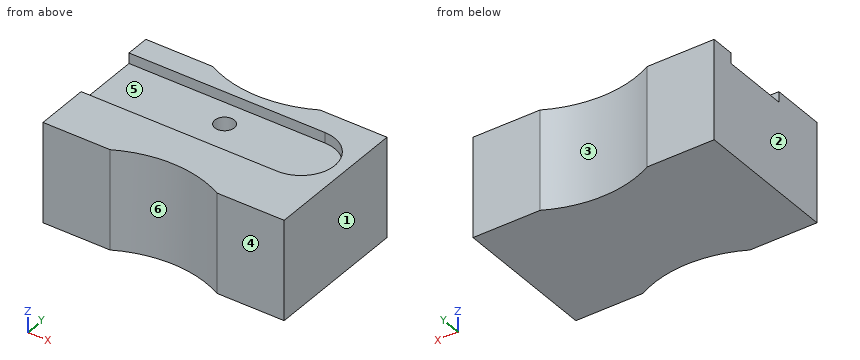
from build123d import *

# Parameters (mm, degrees)
F1_DEPTH = 10.5
F2_DEPTH = 1.1
F3_R     = 1.025
F4_DEPTH = 2.5


with BuildPart() as f1:
    # F0 (on Top) → F1 (new body)
    with BuildSketch(Plane.XY):
        with BuildLine():
            Line((-7.05, 0), (0, 0))
            Line((0, 0), (0, 15.25))
            Line((0, 15.25), (-7.05, 15.25))
            ThreePointArc((-7.05, 15.25), (-12.675, 13.856541), (-18.3, 15.25))
            Line((-18.3, 15.25), (-25.35, 15.25))
            Line((-25.35, 15.25), (-25.35, 12.75))
            Line((-25.35, 12.75), (-4.75, 12.75))
            ThreePointArc((-4.75, 12.75), (-1.2, 9.2), (-4.75, 5.65))
            Line((-4.75, 5.65), (-25.35, 5.65))
            Line((-25.35, 5.65), (-25.35, 0))
            Line((-25.35, 0), (-18.3, 0))
            ThreePointArc((-18.3, 0), (-12.675, 1.393459), (-7.05, 0))
        make_face()
        with BuildLine():
            Line((-25.35, 12.75), (-25.35, 5.65))
            Line((-25.35, 5.65), (-4.75, 5.65))
            ThreePointArc((-4.75, 5.65), (-1.2, 9.2), (-4.75, 12.75))
            Line((-4.75, 12.75), (-25.35, 12.75))
        make_face()
    extrude(amount=-F1_DEPTH)

    # F0 (on Top) → F2 (cut)
    with BuildSketch(Plane.XY):
        with BuildLine():
            Line((-25.35, 12.75), (-25.35, 5.65))
            Line((-25.35, 5.65), (-4.75, 5.65))
            ThreePointArc((-4.75, 5.65), (-1.2, 9.2), (-4.75, 12.75))
            Line((-4.75, 12.75), (-25.35, 12.75))
        make_face()
    extrude(amount=-F2_DEPTH, mode=Mode.SUBTRACT)

    # F3 (on face) → F4 (cut)
    with BuildSketch(Plane.XY.offset(-1.1)):
        with Locations((-13.425, 10.1)):
            Circle(F3_R)
    extrude(amount=-F4_DEPTH, mode=Mode.SUBTRACT)


solid = f1.part
Work out the finished part from the listing and answer in its coordinate system (mm). Face numbers are marked on the shaded views. A direction names the side the tool comes from. Give positions to 0.01 mm unless a question says otherwise; leave off trailing zeros. Loops run counter-clockwise (first coordinate to the right, second up) from the corner with the lowest first, then second, coordinate; pieces in that order, holes last. Notation, with made-up numbers: (48.25, -39) - (82.25, -39) arc R23 cw to (82.25, -19) - close; hole circle Ø7 at (67.5, 77.5). An arc over 180 degrees is marked (long way). Answer in a Markdown table with one row per item. Add a question column.
Q1. The part is cut by section C-C (z = -8.25). Determine the outline of the cut face in (x, y) (3 decimals).
Q2. Consider line 1 along Y through (x, z) = (-6.25, -1); line 2 along Z through (x, y) = (-12.5, 7.5); line 3 along Y through (x, z) = (-12.5, -2.25). Determine where each line is inside the solid, lowest interval first.
Q3. The part is cut by section A-A (z = -2.5). Determine the outline of the cut face in (x, y) (3 decimals), and give its area (3 significant figures).
Q4. Each of these flat-tipped pins is pushed along its axis until it touches: P1, Ø0.6, axis at x = -12, z = -0.5, coming from the +Y side; P2, Ø2, axis at x = -10.5, y = 9, coming from the +Z side; P3, Ø6, axis at x = -13, z = -5, coming from the -Y side. Where does it stop, or does it pass through?
Q5. The part is cut by section B-B (x = -18.75). Determine the outline of the cut face in (y, z), and give its area (3 significant figures).
Q6. The part is cut by section D-D (y = 9.5). Determine the outline of the cut face in (x, z).
Q7. A tool of negligible diameter and unlimited length cuts with its end or side. For the marked faces 5 and 6, from which of +Z, -Z, +X, -X, +Y, -Y can it reach the whole face along a straight path? Write none if from no direction.
Q8. Determine the mould class of the marked faces 1, 2, 3 and 4 for opening direction X: released by +X, released by -X, zero draft, split by the parting line, or undercut.
Solution:
| question | item | result |
|---|---|---|
| 1 | outline | (-25.35, 0) - (-18.3, 0) arc R12.05 cw to (-7.05, 0) - (0, 0) - (0, 15.25) - (-7.05, 15.25) arc R12.05 cw to (-18.3, 15.25) - (-25.35, 15.25) - close |
| 2 | line 1 | y = 0 to 5.65, 12.75 to 15.25 |
| 2 | line 2 | z = -10.5 to -1.1 |
| 2 | line 3 | y = 1.39 to 9.66, 10.54 to 13.86 |
| 3 | outline | (-25.35, 0) - (-18.3, 0) arc R12.05 cw to (-7.05, 0) - (0, 0) - (0, 15.25) - (-7.05, 15.25) arc R12.05 cw to (-18.3, 15.25) - (-25.35, 15.25) - close; hole circle Ø2.05 at (-13.425, 10.1) |
| 3 | area | 362 mm² |
| 4 | P1 | stops at y = 13.9 |
| 4 | P2 | stops at z = -1.1 |
| 4 | P3 | stops at y = 0.93 |
| 5 | outline | (0, -10.5) - (15.25, -10.5) - (15.25, 0) - (12.75, 0) - (12.75, -1.1) - (5.65, -1.1) - (5.65, 0) - (0, 0) - close |
| 5 | area | 152 mm² |
| 6 | outline | (-25.35, -10.5) - (0, -10.5) - (0, 0) - (-1.21, 0) - (-1.21, -1.1) - (-12.59, -1.1) - (-12.59, -3.6) - (-14.26, -3.6) - (-14.26, -1.1) - (-25.35, -1.1) - close |
| 7 | face 5 | +Z, -X |
| 7 | face 6 | +Z, -Z, -Y |
| 8 | face 1 | released by +X |
| 8 | face 2 | released by -X |
| 8 | face 3 | undercut |
| 8 | face 4 | zero draft |
